```python
from build123d import *

# Parameters (mm, degrees)
FILLET1_R   = 0.3
HEX_START   = -2.5
HEX_2_DEPTH = 2.5


with BuildPart() as part:
    # BodySke → BaseBody (revolve)
    with BuildSketch(Plane.XY, mode=Mode.PRIVATE) as basebody_sk:
        Polygon((0, 0), (0, 5.785), (0.515, 5.785), (3.3, 3), (24.4455, 3), (25, 2.4455), (25, 0), align=None)
    revolve(basebody_sk.sketch.rotate(Axis((0, 0, 0), (1, 0, 0)), 90), axis=Axis((0, 0, 0), (1, 0, 0)))

    # Fillet1
    fillet1_edges = [part.edges().sort_by_distance(p)[0] for p in [
        (3.3, 0, -3),
    ]]
    fillet(fillet1_edges, radius=FILLET1_R)

    # Hex 2: read off the stored shape, not the designer's step
    # Hex 2 outline → Hex 2 (cut)
    with BuildSketch(Plane.ZY.offset(HEX_START)):
        Polygon((-2.01, -1.160474041), (0, -2.320948082), (2.01, -1.160474041), (2.01, 1.160474041), (0, 2.320948082), (-2.01, 1.160474041), align=None)
    extrude(amount=HEX_2_DEPTH, mode=Mode.SUBTRACT)

    # Hex 2 2 outline → Hex 2 2 (revolve, cut)
    with BuildSketch(Plane.YX):
        Polygon((2.01, 2.5), (0, 3.660474041), (0, 2.5), align=None)
    revolve(axis=Axis((0, 0, 0), (1, 0, 0)), mode=Mode.SUBTRACT)


solid = part.part
```
CAD build for the part. Positions are in the model's coordinates, mm. A direction names the side the tool comes from. Coordinates: 2 decimals unless noted, no trailing zeros. Order: outer loops, then holes, each group sorted by start corner. A loop starts at its lowest first (then second) coordinate and runs counter-clockwise, first axis right, second up. Notation, with made-up numbers: (30.25, 70) -> (67.25, 70) arc R31 cw to (67.25, 94) -> close; hole circle Ø11 at (0.5, 22). An arc over 180 degrees is marked (long way). Use one line per item in the form item = value. Start each with the question number.
1) Tool access for faces 4 (the flat face through (25, 0, 0)), 5 (the cylindrical face through (14.08, -0.9, 2.86)), 6 (the flat face through (1.27, -1.75, 0.99)): list every direction of +Z, -Z, +X, -X, +Y, -Y with a clear straight run to the whole face (end or side of a thin tool).
2) Band-saw the part on A-A on x = 4.5. Give the cut face in (y, z), then the cut area to 3 significant figures.
3) Pull direction Z, two halves, no side cores. Call faces 1 (the flat face through (0, 2.5, 0.1)), 2 (the flat face through (1, 0, -2.01)), 3 (the conical face through (3.081, 1.233, 2.973)): +Z half, -Z half, draft (parallel to the pull), parting line (faces both ways), or undercut.
4) Drill centre lines: L1, parallel to Z at x = 10, y = 2; L2, parallel to Z at x = 6.25, y = 1.5; L3, parallel to X at y = 1.75, z = -2. Where is each one in solid material? Low to high. Write a range as [from, to].
5) Drop flat-ended pins along their axis: pin 1 (3 mm diameter, centred on y = 2.5, z = -4, fed in from +X); pin 2 (0.7 mm diameter, centred on x = 1.5, y = 0, fed in from -Z); pin 3 (0.5 mm diameter, centred on y = -0.5, z = 1.5, fed in from -X). Give the stop position or say it passes through.
Entries:
q1.face_4 = +Z, -Z, +X, +Y, -Y
q1.face_5 = +X
q1.face_6 = -X
q2.outline = circle Ø6 at (0, 0)
q2.area = 28.3 mm2
q3.face_1 = draft
q3.face_2 = undercut
q3.face_3 = parting line
q4.L1 = [-2.24, 2.24]
q4.L2 = [-2.6, 2.6]
q4.L3 = [0, 24.79]
q5.pin_1 = 3.08
q5.pin_2 = -5.15
q5.pin_3 = 2.6
